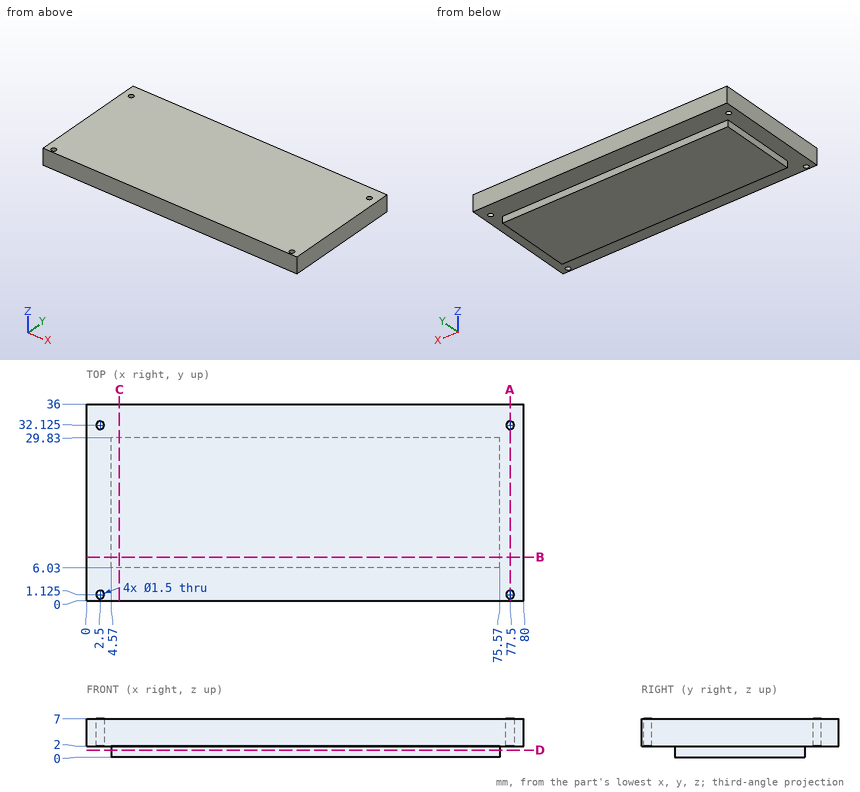
Print and shaded views of the part. All mm, measured from the part's lowest x, y and z. Give positions to 0.01 mm unless a question says otherwise; leave off trailing zeros. Loops run counter-clockwise (first coordinate to the right, second up) from the corner with the lowest first, then second, coordinate; pieces in that order, holes last. Notation, with made-up numbers: (43, 82) - (47, 82) arc R31 cw to (47, 115) - close; hole circle Ø11 at (27.25, 43.25). An arc over 180 degrees is marked (long way). One line per item, written item: value. Start each with the question number.
1. Slice it at D-D (z = 1.25). List the corners of the cut face in (x, y).
2. Slice it at A-A (x = 77.5). List the corners of the cut face in (y, z) (3 decimals).
3. Pin check, flat tips, straight feed: pin 1 (0.6 mm diameter, centred on x = 23, z = 1, fed in from -Y); pin 2 (2 mm diameter, centred on x = 71, z = 5.5, fed in from -Y); pin 3 (1.6 mm diameter, centred on x = 51, z = 1, fed in from +Y); pin 4 (2 mm diameter, centred on x = 77.5, y = 32.125, fed in from -Z). Stop position of each tip, or through.
4. Probe L1, parallel to Y at x = 2.5, z = 5.7 (3 decimals); L2, parallel to X at y = 32.5, z = 6; L3, parallel to Z at x = 58.5, y = 32.5. List the from-to ranges inside material, lowest first. Write a range as from..to.
5. Slice it at B-B (y = 8). List the corners of the cut face in (x, z).
6. Slice it at C-C (x = 6). List the corners of the cut face in (y, z), plus the area to 3 significant figures.
Solution:
1. outline: (4.57, 6.03) - (75.57, 6.03) - (75.57, 29.83) - (4.57, 29.83) - close
2. outline: (0, 2) - (0.375, 2) - (0.375, 7) - (0, 7) - close; (1.875, 2) - (31.375, 2) - (31.375, 7) - (1.875, 7) - close; (32.875, 2) - (36, 2) - (36, 7) - (32.875, 7) - close
3. pin 1: stops at y = 6.03
3. pin 2: stops at y = 0
3. pin 3: stops at y = 29.83
3. pin 4: stops at z = 2
4. L1: y = 0..0.375, 1.875..31.375, 32.875..36
4. L2: x = 0..1.85, 3.15..76.85, 78.15..80
4. L3: z = 2..7
5. outline: (0, 2) - (4.57, 2) - (4.57, 0) - (75.57, 0) - (75.57, 2) - (80, 2) - (80, 7) - (0, 7) - close
6. outline: (0, 2) - (6.03, 2) - (6.03, 0) - (29.83, 0) - (29.83, 2) - (36, 2) - (36, 7) - (0, 7) - close
6. area: 228 mm^2
